Could you check a few things on this model? Use its own coordinates, in mm. A direction names the side the tool comes from. Round coordinates to 2 decimals unless told otherwise and drop trailing zeros. Write each loop counter-clockwise with the first axis right and the second up, starting at its lowest first coordinate (ties: lowest second). Pieces come first, ordered by that corner, then holes. Notation, with made-up numbers: (-39, 1) -> (-33, 1) arc R24 cw to (-33, 32) -> close; hole circle Ø2 at (59.25, 27.5). An arc over 180 degrees is marked (long way). Answer in a Markdown table with one row per item.
from build123d import *

# Parameters (mm, degrees)
SKETCH_1_R          = 11
EXTRUDE_1_DEPTH     = 2
SKETCH_2_R          = 10
EXTRUDE_2_DEPTH     = 6
SKETCH_3_R          = 8.5
EXTRUDE_3_DEPTH     = 17
CUT_EXTRUDE_1_DEPTH = 2
CUT_EXTRUDE_2_DEPTH = 30.444863729
SKETCH_6_W          = 1
SKETCH_6_H          = 0.8
CHAMFER_1_SIZE      = 0.5
SKETCH_8_R          = 7.5
CUT_EXTRUDE_4_DEPTH = 5


with BuildPart() as part:
    # Sketch 1 → Extrude 1 (new body)
    with BuildSketch(Plane(origin=(0, 0, 0), x_dir=(0, 0, -1), z_dir=(1, 0, 0))):
        Circle(SKETCH_1_R)
    extrude(amount=EXTRUDE_1_DEPTH)

    # Sketch 2 → Extrude 2 (add)
    with BuildSketch(Plane(origin=(2, 0, 0), x_dir=(0, 0, -1), z_dir=(1, 0, 0))):
        Circle(SKETCH_2_R)
    extrude(amount=EXTRUDE_2_DEPTH)

    # Sketch 3 → Extrude 3 (add)
    with BuildSketch(Plane(origin=(8, 0, 0), x_dir=(0, 0, -1), z_dir=(1, 0, 0))):
        Circle(SKETCH_3_R)
    extrude(amount=EXTRUDE_3_DEPTH)

    # Sketch 4 → Cut-Extrude 1 (cut)
    with BuildSketch(Plane(origin=(0, 8.5, 0), x_dir=(1, 0, 0), z_dir=(0, 1, 0))):
        with BuildLine():
            Line((10.5, 2), (14.5, 2))
            ThreePointArc((14.5, 2), (16.5, 0), (14.5, -2))
            Line((14.5, -2), (10.5, -2))
            ThreePointArc((10.5, -2), (8.5, 0), (10.5, 2))
        make_face()
    extrude(amount=-CUT_EXTRUDE_1_DEPTH, mode=Mode.SUBTRACT)

    # Sketch 5 → Cut-Extrude 2 (cut, through all)
    with BuildSketch(Plane(origin=(25, 0, 0), x_dir=(0, 0, -1), z_dir=(1, 0, 0))):
        with BuildLine():
            Line((-3, 4), (3, 4))
            ThreePointArc((3, 4), (0, -5), (-3, 4))
        make_face()
    extrude(amount=-CUT_EXTRUDE_2_DEPTH, mode=Mode.SUBTRACT)

    # Sketch 6 → Cut-Revolve 1 (revolve, cut)
    with BuildSketch(Plane.XY, mode=Mode.PRIVATE) as cut_revolve_1_sk:
        with Locations((23.5, 8.5)):
            Rectangle(SKETCH_6_W, SKETCH_6_H)
    revolve(cut_revolve_1_sk.sketch.rotate(Axis((0, 0, 0), (1, 0, 0)), 90), axis=Axis((0, 0, 0), (1, 0, 0)), mode=Mode.SUBTRACT)

    # Chamfer 1
    chamfer_1_edges = [part.edges().sort_by_distance(p)[0] for p in [
        (25, 0, 8.5),
    ]]
    chamfer(chamfer_1_edges, length=CHAMFER_1_SIZE)

    # Sketch 8 → Cut-Extrude 4 (cut)
    with BuildSketch(Plane.ZY):
        Circle(SKETCH_8_R)
    extrude(amount=-CUT_EXTRUDE_4_DEPTH, mode=Mode.SUBTRACT)


solid = part.part
1) Thinking about a two-plate mould opening in Y: for faces 5 (the face through (0, 2.6, -7.2)), 6 (the face through (4.96, -9.76, 2.17)), 7 (the face through (15, 4, 0)), which applies, +Y half, -Y half, draft (parallel to the pull), parting line (faces both ways), or undercut?
Findings:
| item | result |
|---|---|
| face 5 | draft |
| face 6 | parting line |
| face 7 | undercut |
2) Imagine slicing it at D-D, the plane x = 15. Please give me the cut outline in (y, z), plus the area to 3 significant figures.
Findings:
| item | result |
|---|---|
| outline | (6.5, -1.94) -> (6.5, 1.94) -> (8.28, 1.94) arc R8.5 ccw (long way) to (8.28, -1.94) -> close; hole (4, -3) -> (4, 3) arc R5 ccw (long way) to start |
| area | 145 mm^2 |
3) Imagine slicing it at C-C, the plane x = 18. Please give me the cut outline in (y, z), plus the area to 3 significant figures.
Findings:
| item | result |
|---|---|
| outline | circle Ø17 at (0, 0); hole (4, -3) -> (4, 3) arc R5 ccw (long way) to start |
| area | 153 mm^2 |
4) Imagine slicing it at B-B, the plane x = 12.5. Please give me the cut outline in (y, z), plus the area to 3 significant figures.
Findings:
| item | result |
|---|---|
| outline | (6.5, -2) -> (6.5, 2) -> (8.26, 2) arc R8.5 ccw (long way) to (8.26, -2) -> close; hole (4, -3) -> (4, 3) arc R5 ccw (long way) to start |
| area | 145 mm^2 |
5) Please list where these lines run through material, in increasing order: line 1 (Y direction, x = 2.7, z = 0); line 2 (Z direction, x = 17.25, y = 0); line 3 (Y direction, x = 1.75, z = 0).
Findings:
| item | result |
|---|---|
| line 1 | y = -10 to -7.5, 7.5 to 10 |
| line 2 | z = -8.5 to -5, 5 to 8.5 |
| line 3 | y = -11 to -7.5, 7.5 to 11 |
6) For pin 1 (12 mm diameter, centred on x = 21, z = 2, fed in from +Y); pin 2 (3 mm diameter, centred on x = 20, y = 1, fed in from -Z); pin 3 (11.5 mm diameter, centred on y = 0, z = 0, fed in from -X), each with a flat end and sliding along its axis, tell me the tip position at first contact or that it passes through.
Findings:
| item | result |
|---|---|
| pin 1 | stops at y = 8.5 |
| pin 2 | stops at z = -8.5 |
| pin 3 | stops at x = 5 |
7) For faces 1 (the face through (13, 7, 2)), 2 (the face through (23.507, 7.907, -1.756)), 3 (the face through (2, -10, -2)), 4 (the face through (5, -5, 2)), which set-ups out of +Z, -Z, +X, -X, +Y, -Y let a thin tool reach every point of the face, with its end or its side?
Findings:
| item | result |
|---|---|
| face 1 | +Y |
| face 2 | none |
| face 3 | +X |
| face 4 | -X |
